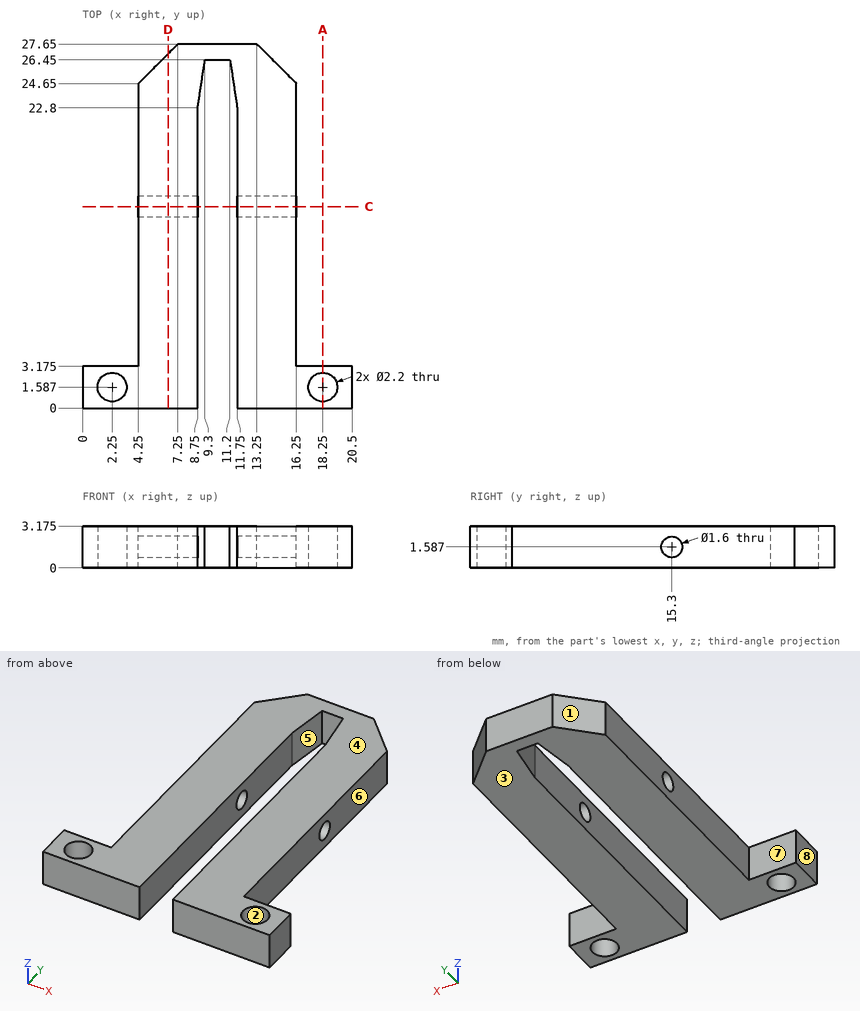
Geometry: see drawing. Coordinates: mm, zero at the bounding-box minimum. A direction names the side the tool comes from. Coordinates: 2 decimals unless noted, no trailing zeros. Loops run counter-clockwise (first coordinate to the right, second up) from the corner with the lowest first, then second, coordinate; pieces in that order, holes last. Notation, with made-up numbers: (48.5, -7.5) - (76.5, -7.5) arc R19 ccw to (76.5, 17.5) - close; hole circle Ø9 at (85.25, 28). An arc over 180 degrees is marked (long way). Put each result on its own line as item: value. Start each with the question number.
Q1. Cut plane C-C, the plane y = 15.3. Give the number of separate pieces and of enclosed holes in the cut face.
Q2. Cut plane D-D, the plane x = 6.5. Return loops of the section in (y, z) (1 decimal).
Q3. Pin query (flat end, axial travel): pin 1 Ø1 at (x, z) = (18.5, 1) entering from +Y (1 decimal); pin 2 Ø1 at (y, z) = (17, 2) entering from +X; pin 3 Ø1 at (x, z) = (15, 2) entering from +Y. Return the tip coordinate at first contact, or that it passes through.
Q4. Cut plane A-A, the plane x = 18.25. Return loops of the section in (y, z) (1 decimal).
Q5. Pull-direction query (Y, two-part tool) for the marked faces 1, 2 and 3; classes: released by +Y, released by -Y, zero draft, split by the parting line, or undercut.
Q6. Set-up query: the marked faces 4, 5, 6, 7 and 8. Return all of +Z, -Z, +X, -X, +Y, -Y with unobstructed straight access to the full face (end or side cutting, diameter ignored); none if empty.
Q7. Line query: line 1 (Y direction, x = 2.25, z = 0.8) (1 decimal); line 2 (Y direction, x = 19, z = 0.8) (1 decimal); line 3 (X direction, y = 7.5, z = 0.7). Output: solid intervals per line, ascending.
Filled sheet:
1. separate pieces: 4
1. enclosed holes: 0
2. outline: (0, 0) - (26.9, 0) - (26.9, 3.2) - (0, 3.2) - close; hole circle Ø1.6 at (15.3, 1.6)
3. pin 1: y = 3.2
3. pin 2: x = 16.25
3. pin 3: y = 26.4
4. outline: (0, 0) - (0.5, 0) - (0.5, 3.2) - (0, 3.2) - close; (2.7, 0) - (3.2, 0) - (3.2, 3.2) - (2.7, 3.2) - close
5. face 1: released by +Y
5. face 2: undercut
5. face 3: zero draft
6. face 4: +Z, +X, -X, +Y, -Y
6. face 5: +Z, -Z, -Y
6. face 6: +Z, -Z, +X, +Y
6. face 7: +Z, -Z, -X, +Y
6. face 8: +Z, -Z, -X, +Y, -Y
7. line 1: 0 to 0.5, 2.7 to 3.2
7. line 2: 0 to 0.8, 2.4 to 3.2
7. line 3: 4.25 to 8.75, 11.75 to 16.25
